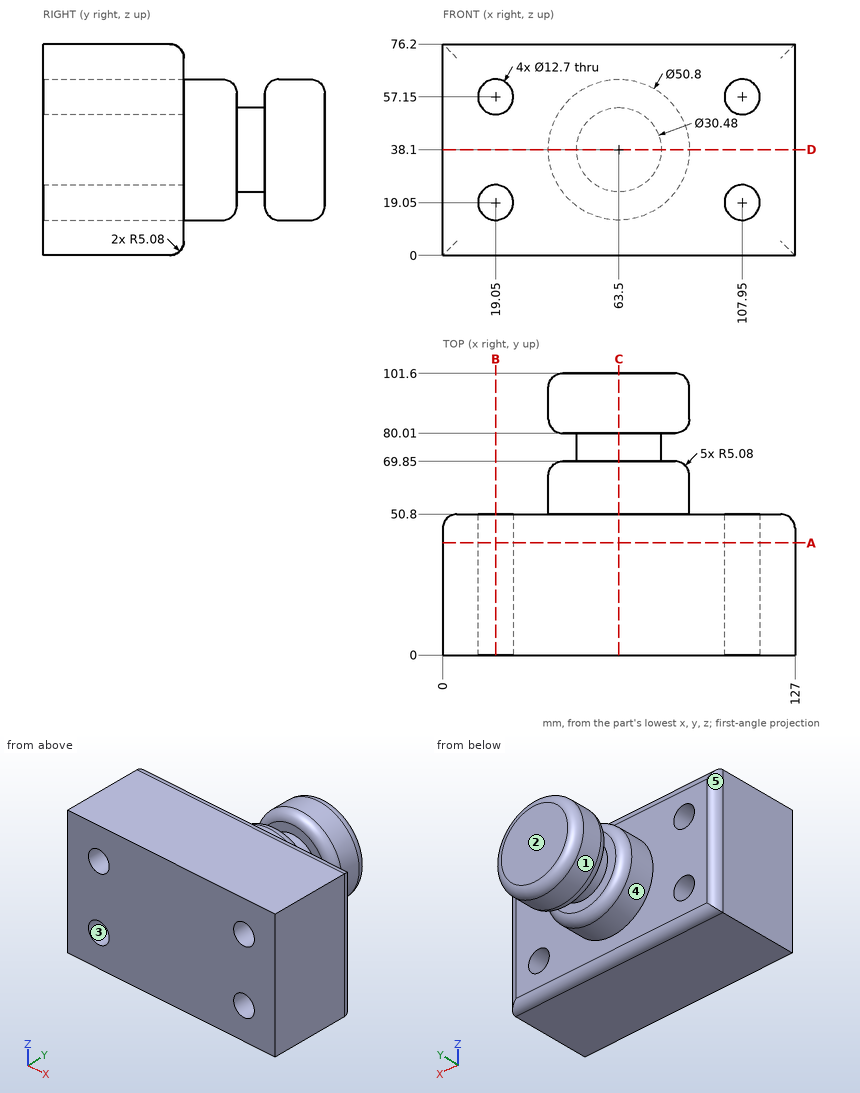
Verification items for this drawing (mm, ordinates from the low corner). A direction names the side the tool comes from. Give positions to 0.01 mm unless a question says otherwise; leave off trailing zeros. Loops run counter-clockwise (first coordinate to the right, second up) from the corner with the lowest first, then second, coordinate; pieces in that order, holes last. Notation, with made-up numbers: M 28,-20.75 L 47,-20.75 A29 cw 47,1.25 Z; hole C -33,20 d9. An arc over 180 degrees is marked long. Answer as a JSON object with one key per item and string values. Group by question number.
Item 1: Sectioned sample at B-B on x = 19.05. Record the boundary of the cut face in (y, z), plus the area to 3 significant figures.
Item 2: Gauge pin test, flat ends, axial feed: pin 1 (7.5 mm diameter, centred on x = 19.05, z = 57.15, fed in from -Y); pin 2 (4 mm diameter, centred on y = 72, z = 53.5, fed in from +X); pin 3 (12 mm diameter, centred on x = 48, y = 75.5, fed in from +Z); pin 4 (4 mm diameter, centred on x = 15, z = 40, fed in from +Y). Record the tip position at first contact, or that the pin passes through.
Item 3: Sectioned sample at C-C on x = 63.5. Record the boundary of the cut face in (y, z).
Item 4: Sectioned sample at A-A on y = 40.5. Record the boundary of the cut face in (x, z), plus the area to 3 significant figures.
Item 5: Material ranges on L1, parallel to Z at x = 19.05, y = 12.5; L2, parallel to X at y = 20, z = 19; L3, parallel to Y at x = 48, z = 31.5, recorded low to high.
Item 6: Mould release check, pull along X, two halves, no side actions. Record for the marked faces 3, 4 and 5: pulls with the +X half, pulls with the -X half, needs draft (parallel to the pull), parting line crosses it, or undercut.
Item 7: Sectioned sample at D-D on z = 38.1. Record the boundary of the cut face in (x, y), plus the area to 3 significant figures.
Item 8: Access from +Z, -Z, +X, -X, +Y, -Y to the whole of each face (thin tool, end or side, straight path). Record for the marked faces 1 and 2.
Findings below:
{
 "1": {"outline": "M 0,0 L 45.72,0 A5.08 ccw 50.8,5.08 L 50.8,12.7 L 0,12.7 Z; M 0,25.4 L 50.8,25.4 L 50.8,50.8 L 0,50.8 Z; M 0,63.5 L 50.8,63.5 L 50.8,71.12 A5.08 ccw 45.72,76.2 L 0,76.2 Z", "area": "2,570 mm2"},
 "2": {"pin 1": "through", "pin 2": "x = 70.76", "pin 3": "z = 57.41", "pin 4": "y = 50.8"},
 "3": {"outline": "M 0,0 L 45.72,0 A5.08 ccw 50.8,5.08 L 50.8,12.7 L 64.77,12.7 A5.08 ccw 69.85,17.78 L 69.85,22.86 L 80.01,22.86 L 80.01,17.78 A5.08 ccw 85.09,12.7 L 96.52,12.7 A5.08 ccw 101.6,17.78 L 101.6,58.42 A5.08 ccw 96.52,63.5 L 85.09,63.5 A5.08 ccw 80.01,58.42 L 80.01,53.34 L 69.85,53.34 L 69.85,58.42 A5.08 ccw 64.77,63.5 L 50.8,63.5 L 50.8,71.12 A5.08 ccw 45.72,76.2 L 0,76.2 Z"},
 "4": {"outline": "M 0,0 L 127,0 L 127,76.2 L 0,76.2 Z; hole C 19.05,19.05 d12.7; hole C 19.05,57.15 d12.7; hole C 107.95,19.05 d12.7; hole C 107.95,57.15 d12.7", "area": "9,170 mm2"},
 "5": {"L1": "0 to 12.7, 25.4 to 50.8, 63.5 to 76.2", "L2": "0 to 12.7, 25.4 to 101.6, 114.3 to 127", "L3": "0 to 69.85, 80.01 to 101.6"},
 "6": {"face 3": "undercut", "face 4": "parting line crosses it", "face 5": "pulls with the -X half"},
 "7": {"outline": "M 0,0 L 127,0 L 127,45.72 A5.08 ccw 121.92,50.8 L 88.9,50.8 L 88.9,64.77 A5.08 ccw 83.82,69.85 L 78.74,69.85 L 78.74,80.01 L 83.82,80.01 A5.08 ccw 88.9,85.09 L 88.9,96.52 A5.08 ccw 83.82,101.6 L 43.18,101.6 A5.08 ccw 38.1,96.52 L 38.1,85.09 A5.08 ccw 43.18,80.01 L 48.26,80.01 L 48.26,69.85 L 43.18,69.85 A5.08 ccw 38.1,64.77 L 38.1,50.8 L 5.08,50.8 A5.08 ccw 0,45.72 Z", "area": "8,780 mm2"},
 "8": {"face 1": "+Y", "face 2": "+Z, -Z, +X, -X, +Y"}
}
